The drawing under review shows one solid part. Ordinate dimensions are in mm from its lowest x, y, z. Coordinates: 2 decimals unless noted, no trailing zeros. Write each loop counter-clockwise with the first axis right and the second up, starting at its lowest first coordinate (ties: lowest second). Pieces come first, ordered by that corner, then holes.
1) We need section D-D on y = 25.4. Write out the cut boundary in (x, z), then the cut area to 3 significant figures.
2) We need section A-A on y = 64. Write out the cut boundary in (x, z).
3) To check wall thickness, follow line 1 along Y through (x, z) = (38.1, 1.35); line 2 along X through (y, z) = (38, 1.9); line 3 along Y through (x, z) = (12.7, 3.1). State the ranges of each line that lie inside material, in increasing order.
4) We need section B-B on z = 2.65. Write out the cut boundary in (x, y).
5) Insertion check: P1, Ø3, axis at x = 12.7, y = 25.4, coming from the +Z side. The pin has a flat end and moves straight along its axis. Give the tip position at first contact, or say it passes through.
6) We need section C-C on x = 63.5. Write out the cut boundary in (y, z).
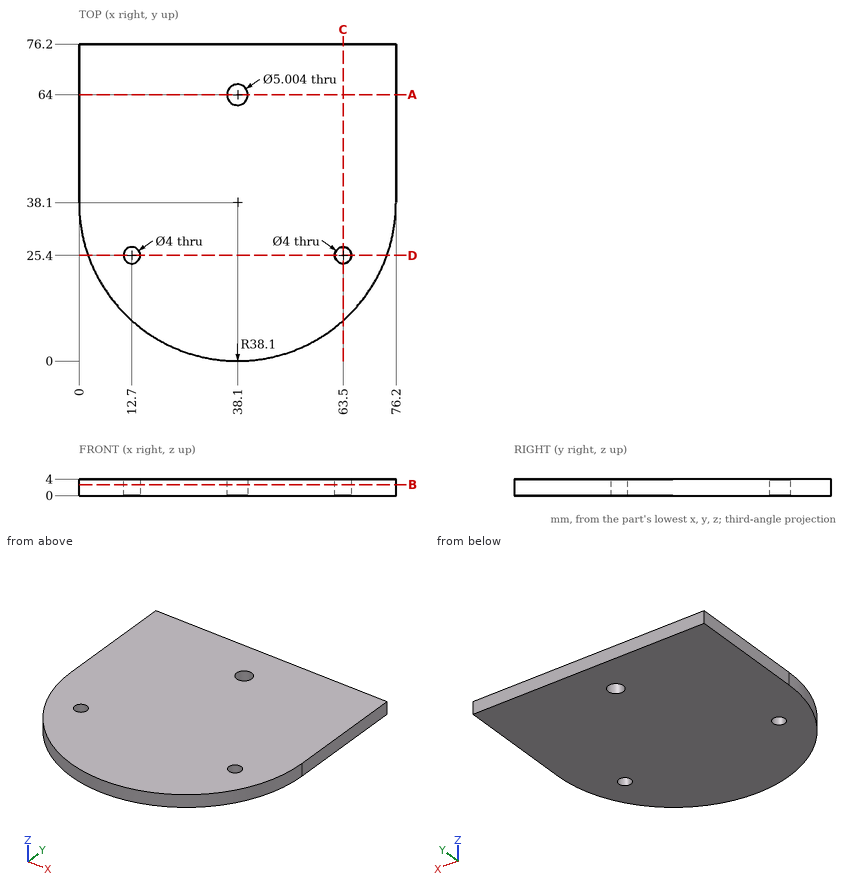
Result:
1. outline: (2.18, 0) - (10.7, 0) - (10.7, 4) - (2.18, 4) - close; (14.7, 0) - (61.5, 0) - (61.5, 4) - (14.7, 4) - close; (65.5, 0) - (74.02, 0) - (74.02, 4) - (65.5, 4) - close
1. area: 255 mm2
2. outline: (0, 0) - (35.6, 0) - (35.6, 4) - (0, 4) - close; (40.6, 0) - (76.2, 0) - (76.2, 4) - (40.6, 4) - close
3. line 1: y = 0 to 61.5, 66.5 to 76.2
3. line 2: x = 0 to 76.2
3. line 3: y = 9.7 to 23.4, 27.4 to 76.2
4. outline: (0, 38.1) arc R38.1 ccw to (76.2, 38.1) - (76.2, 76.2) - (0, 76.2) - close; hole circle Ø4 at (12.7, 25.4); hole circle Ø5 at (38.1, 64); hole circle Ø4 at (63.5, 25.4)
5. P1: passes through
6. outline: (9.7, 0) - (23.4, 0) - (23.4, 4) - (9.7, 4) - close; (27.4, 0) - (76.2, 0) - (76.2, 4) - (27.4, 4) - close
